Geometry: final body of the model. Coordinates: model frame, mm. A direction names the side the tool comes from. Give positions to 0.01 mm unless a question says otherwise; leave off trailing zeros. Write each loop counter-clockwise with the first axis right and the second up, starting at its lowest first coordinate (ties: lowest second). Pieces come first, ordered by that corner, then holes. Notation, with made-up numbers: M 74,-22 L 96,-22 A7 ccw 96,-14 Z; hole C 64.5,30.25 d4. An arc over 180 degrees is marked long. Answer as a JSON object with one key per item and string values.
from build123d import *

# Parameters (mm, degrees)
BOSS_EXTRUDE1_DEPTH = 10
SKETCH2_R           = 23.5
CUT_EXTRUDE1_DEPTH  = 2.5
SKETCH4_R           = 8
CUT_EXTRUDE3_DEPTH  = 104.047319228
BOSS_EXTRUDE3_START = 50
BOSS_EXTRUDE3_DEPTH = 50
SKETCH8_R           = 1.5
CUT_EXTRUDE4_DEPTH  = 10
SKETCH9_R           = 4
CUT_EXTRUDE5_DEPTH  = 120.006302354
SKETCH10_R          = 10
CUT_EXTRUDE6_DEPTH  = 5
SKETCH11_R          = 2.5
CUT_EXTRUDE7_DEPTH  = 120.006302354


with BuildPart() as part:
    # Sketch1 → Boss-Extrude1 (new body)
    with BuildSketch(Plane(origin=(0, 0, 0), x_dir=(1, 0, 0), z_dir=(0, 1, 0))):
        with BuildLine():
            Line((-32.5, 65), (-32.5, -65))
            ThreePointArc((-32.5, -65), (0, -97.5), (32.5, -65))
            Line((32.5, -65), (32.5, 65))
            ThreePointArc((32.5, 65), (0, 97.5), (-32.5, 65))
        make_face()
    extrude(amount=BOSS_EXTRUDE1_DEPTH)

    # Sketch2 → Cut-Extrude1 (cut)
    with BuildSketch(Plane(origin=(0, 10, 0), x_dir=(1, 0, 0), z_dir=(0, 1, 0))):
        with Locations(Location((0, 65, 0), (0, 0, 270))):
            Circle(SKETCH2_R)
    extrude(amount=-CUT_EXTRUDE1_DEPTH, mode=Mode.SUBTRACT)

    # Sketch4 → Cut-Extrude3 (cut, through all)
    with BuildSketch(Plane(origin=(0, 7.5, 0), x_dir=(1, 0, 0), z_dir=(0, 1, 0))):
        with Locations(Location((0, 65, 0), (0, 0, 270))):
            Circle(SKETCH4_R)
    extrude(amount=-CUT_EXTRUDE3_DEPTH, mode=Mode.SUBTRACT)

    # Sketch7 → Boss-Extrude3 (add)
    with BuildSketch(Plane.XZ.offset(BOSS_EXTRUDE3_START)):
        with BuildLine():
            Line((-30.5, 65), (-32.5, 65))
            ThreePointArc((-32.5, 65), (0, 97.5), (32.5, 65))
            Line((32.5, 65), (30.5, 65))
            ThreePointArc((30.5, 65), (0, 95.5), (-30.5, 65))
        make_face()
        with BuildLine():
            Line((-32.5, -65), (-30.5, -65))
            ThreePointArc((-30.5, -65), (0, -95.5), (30.5, -65))
            Line((30.5, -65), (32.5, -65))
            ThreePointArc((32.5, -65), (0, -97.5), (-32.5, -65))
        make_face()
    extrude(amount=-BOSS_EXTRUDE3_DEPTH)

    # Sketch8 → Cut-Extrude4 (cut)
    with BuildSketch(Plane(origin=(0, 7.5, 0), x_dir=(1, 0, 0), z_dir=(0, 1, 0))):
        with Locations(Location((13.5, 65, 0), (0, 0, 270))):
            Circle(SKETCH8_R)
        with Locations(Location((0, 78.5, 0), (0, 0, 270))):
            Circle(SKETCH8_R)
        with Locations(Location((-13.5, 65, 0), (0, 0, 270))):
            Circle(SKETCH8_R)
        with Locations(Location((0, 51.5, 0), (0, 0, 270))):
            Circle(SKETCH8_R)
    extrude(amount=-CUT_EXTRUDE4_DEPTH, mode=Mode.SUBTRACT)

    # Sketch9 → Cut-Extrude5 (cut, through all)
    with BuildSketch(Plane(origin=(0, 10, 0), x_dir=(1, 0, 0), z_dir=(0, 1, 0))):
        with Locations(Location((0, -65, 0), (0, 0, 270))):
            Circle(SKETCH9_R)
    extrude(amount=-CUT_EXTRUDE5_DEPTH, mode=Mode.SUBTRACT)

    # Sketch10 → Cut-Extrude6 (cut)
    with BuildSketch(Plane(origin=(0, 10, 0), x_dir=(1, 0, 0), z_dir=(0, 1, 0))):
        with Locations(Location((0, -65, 0), (0, 0, 270))):
            Circle(SKETCH10_R)
    extrude(amount=-CUT_EXTRUDE6_DEPTH, mode=Mode.SUBTRACT)

    # Sketch11 → Cut-Extrude7 (cut, through all)
    with BuildSketch(Plane(origin=(0, 10, 0), x_dir=(1, 0, 0), z_dir=(0, 1, 0))):
        with Locations(Location((-26, 32.5, 0), (0, 0, 270))):
            Circle(SKETCH11_R)
        with Locations(Location((26, 32.5, 0), (0, 0, 270))):
            Circle(SKETCH11_R)
    extrude(amount=-CUT_EXTRUDE7_DEPTH, mode=Mode.SUBTRACT)


solid = part.part
1) Cut plane C-C on z = -71. Return loops of the section in (x, y).
Geometry check:
{"outline": "M -31.94,-50 L -29.9,-50 L -29.9,0 L -5.29,0 L -5.29,7.5 L -22.72,7.5 L -22.72,10 L -31.94,10 Z; M 5.29,0 L 29.9,0 L 29.9,-50 L 31.94,-50 L 31.94,10 L 22.72,10 L 22.72,7.5 L 5.29,7.5 Z"}
2) Cut plane A-A on y = -4.5. Return loops of the section in (x, z).
Geometry check:
{"outline": "M -32.5,-65 A32.5 ccw 32.5,-65 L 30.5,-65 A30.5 cw -30.5,-65 Z; M -32.5,65 L -30.5,65 A30.5 cw 30.5,65 L 32.5,65 A32.5 ccw Z"}
3) Set-up query: faces 4 (the cylindrical face through (1.033, 8.768, -88.477)), 5 (the cylindrical face through (-0.715, -20.42, 97.492)), 6 (the cylindrical face through (0.671, -25.35, 95.493)). Return all of +Z, -Z, +X, -X, +Y, -Y with unobstructed straight access to the full face (end or side cutting, diameter ignored); none if empty.
Geometry check:
{"face 4": "+Y", "face 5": "+Z, +Y, -Y", "face 6": "-Y"}
4) Line query: line 1 (X direction, y = 3.25, z = -32.5); line 2 (X direction, y = 2.5, z = -65); line 3 (Y direction, x = 10, z = 59). Output: solid intervals per line, ascending. Write a range as from..to.
Geometry check:
{"line 1": "x = -32.5..-28.5, -23.5..23.5, 28.5..32.5", "line 2": "x = -32.5..-15, -12..-8, 8..12, 15..32.5", "line 3": "y = 0..10"}
5) Cut plane B-B on z = -32.5. Return loops of the section in (x, y), and give its area (3 significant figures).
Geometry check:
{"outline": "M -32.5,0 L -28.5,0 L -28.5,10 L -32.5,10 Z; M -23.5,0 L 23.5,0 L 23.5,10 L -23.5,10 Z; M 28.5,0 L 32.5,0 L 32.5,10 L 28.5,10 Z", "area": "550 mm2"}
6) Contact query for flat-ended pins moving along their axis: P1, Ø2, axis at x = 1, z = 63, coming from the -Y side; P2, Ø4, axis at x = 5, z = -13.5, coming from the -Y side; P3, Ø4, axis at x = 0, z = -78.5, coming from the +Y side; P4, Ø6.5, axis at x = 26, z = -32.5, coming from the +Y side. Output: stop coordinate, or through.
Geometry check:
{"P1": "passes through", "P2": "stops at y = 0", "P3": "stops at y = 7.5", "P4": "stops at y = 10"}
7) Pull-direction query (X, two-part tool) for faces 1 (the flat face through (0, -50, 96)), 2 (the flat face through (32.5, 5, 1)), 3 (the flat face through (0, 7.5, -55)); classes: pulls with the +X half, pulls with the -X half, needs draft (parallel to the pull), parting line crosses it, or undercut.
Geometry check:
{"face 1": "needs draft", "face 2": "pulls with the +X half", "face 3": "undercut"}
8) Cut plane D-D on x = -21. Return loops of the section in (y, z), and give its area (3 significant figures).
Geometry check:
{"outline": "M -50,-89.8 L 10,-89.8 L 10,-75.55 L 7.5,-75.55 L 7.5,-54.45 L 10,-54.45 L 10,89.8 L -50,89.8 L -50,87.12 L 0,87.12 L 0,-87.12 L -50,-87.12 Z", "area": "2,010 mm2"}
